Design review of the part built by this model. Coordinates are the model's own, in mm. A direction names the side the tool comes from. Round coordinates to 2 decimals unless told otherwise and drop trailing zeros. Write each loop counter-clockwise with the first axis right and the second up, starting at its lowest first coordinate (ties: lowest second). Pieces come first, ordered by that corner, then holes. Notation, with made-up numbers: M 0.25,-12.5 L 47.25,-12.5 A14 cw 47.25,13.5 Z; hole C 7,-27.5 d8. An arc over 180 degrees is marked long. One line per question, with ' | ' between items. Start each with the question number.
Item 1: Add section D-D, the plane z = 5. State the section outline as (x, y) points.
Item 2: Add section C-C, the plane z = 28.5. State the section outline as (x, y) points.
Item 3: Draft analysis for pull direction Z (two halves, no side actions). For faces 5 (the face through (60, 99, 20)), 6 (the face through (39.08, 42.535, 22.365)), 7 (the face through (21.6, 99.5, 2)), 8 (the face through (-1, 55, 0)), state which applies: released by +Z, released by -Z, zero draft, split by the parting line, or undercut.
Item 4: For L1, parallel to Z at x = -15.5, y = 3.8; L2, parallel to X at y = 100.4, z = 5; L3, parallel to Y at x = 45, z = 11, list the stretches that pass through material, from the lowest coordinate up.
Item 5: Machinability: for faces 1 (the face through (0, 20, 20)), 2 (the face through (3.57, 42.46, 4.35)), 3 (the face through (54.474, 99.535, 4.609)), 4 (the face through (30, 97, 20)), which of the approach directions +Z, -Z, +X, -X, +Y, -Y give a long, thin tool a straight path to every point of the face, cutting with its end or side? Answer none if there is none.
Item 6: Add section A-A, the plane x = 6.5. State the section outline as (y, z) points, and give its area (3 significant figures).
Item 7: Insertion check: pin 1 Ø9.5 at (x, z) = (36.5, 20) entering from +Y; pin 2 Ø4 at (x, z) = (-15.5, 11.5) entering from -Y; pin 3 Ø10 at (x, z) = (16, 6.5) entering from -Y; pin 4 Ø13.5 at (x, z) = (-19, 18) entering from +Y. Each pin has a flat end and moves straight along its axis. Give the tip position at first contact, or say it passes through.
Item 8: Add section B-B, the plane x = 36.5. State the section outline as (y, z) points.
```python
from build123d import *

# Parameters (mm, degrees)
SALIENTE_EXTRUIR1_DEPTH = 40
CORTAR_EXTRUIR1_REACH   = 122.868
CROQUIS2_R              = 3.5
CORTAR_EXTRUIR4_START   = -62
CROQUIS3_R              = 3
CORTAR_EXTRUIR4_DEPTH   = 5
CORTAR_EXTRUIR3_REACH   = 93.918
CROQUIS4_R              = 2.5
CROQUIS4_R_2            = 3.5
CORTAR_EXTRUIR5_REACH   = 126.916
CROQUIS5_R              = 3


with BuildPart() as part:
    # Croquis1 → Saliente-Extruir1 (new body)
    with BuildSketch(Plane.XY):
        Polygon((0, 0), (0, 40), (60, 40), (60, 45), (0, 45), (0, 97), (60, 97), (60, 102), (-7, 102), (-7, 5), (-24, 5), (-24, 0), align=None)
    extrude(amount=SALIENTE_EXTRUIR1_DEPTH)

    # Croquis2 → Cortar-Extruir1 (cut, up to next)
    with BuildSketch(Plane(origin=(0, 5, 0), x_dir=(1, 0, 0), z_dir=(0, 1, 0)), mode=Mode.PRIVATE) as cortar_extruir1_sk1:
        with Locations(Location((-15.5, -11.5, 0), (0, 0, 180))):
            Circle(CROQUIS2_R)
    cortar_extruir1_tool1 = extrude(cortar_extruir1_sk1.sketch, amount=-CORTAR_EXTRUIR1_REACH, mode=Mode.PRIVATE) & part.part
    # Croquis2 → Cortar-Extruir1 (cut, up to next)
    with BuildSketch(Plane(origin=(0, 5, 0), x_dir=(1, 0, 0), z_dir=(0, 1, 0)), mode=Mode.PRIVATE) as cortar_extruir1_sk2:
        with Locations(Location((-15.5, -28.5, 0), (0, 0, 180))):
            Circle(CROQUIS2_R)
    cortar_extruir1_tool2 = extrude(cortar_extruir1_sk2.sketch, amount=-CORTAR_EXTRUIR1_REACH, mode=Mode.PRIVATE) & part.part
    add(cortar_extruir1_tool1.solids().sort_by_distance((-15.5, 5, 11.5))[0], mode=Mode.SUBTRACT)
    add(cortar_extruir1_tool2.solids().sort_by_distance((-15.5, 5, 28.5))[0], mode=Mode.SUBTRACT)

    # Croquis3 → Cortar-Extruir4 (cut)
    with BuildSketch(Plane(origin=(0, 102, 0), x_dir=(1, 0, 0), z_dir=(0, 1, 0)).offset(CORTAR_EXTRUIR4_START)):
        with Locations(Location((6.5, -5, 0), (0, 0, 270))):
            Circle(CROQUIS3_R)
        with Locations(Location((36.5, -5, 0), (0, 0, 270))):
            Circle(CROQUIS3_R)
        with Locations(Location((6.5, -35, 0), (0, 0, 270))):
            Circle(CROQUIS3_R)
        with Locations(Location((36.5, -35, 0), (0, 0, 270))):
            Circle(CROQUIS3_R)
    extrude(amount=CORTAR_EXTRUIR4_DEPTH, mode=Mode.SUBTRACT)

    # Croquis4 → Cortar-Extruir3 (cut, up to next)
    with BuildSketch(Plane(origin=(0, 45, 0), x_dir=(1, 0, 0), z_dir=(0, 1, 0)), mode=Mode.PRIVATE) as cortar_extruir3_sk1:
        with Locations(Location((21.5, -20, 0), (0, 0, 180))):
            Circle(CROQUIS4_R)
    cortar_extruir3_tool1 = extrude(cortar_extruir3_sk1.sketch, amount=-CORTAR_EXTRUIR3_REACH, mode=Mode.PRIVATE) & part.part
    # Croquis4 → Cortar-Extruir3 (cut, up to next)
    with BuildSketch(Plane(origin=(0, 45, 0), x_dir=(1, 0, 0), z_dir=(0, 1, 0)), mode=Mode.PRIVATE) as cortar_extruir3_sk2:
        with Locations(Location((36.5, -20, 0), (0, 0, 180))):
            Circle(CROQUIS4_R_2)
    cortar_extruir3_tool2 = extrude(cortar_extruir3_sk2.sketch, amount=-CORTAR_EXTRUIR3_REACH, mode=Mode.PRIVATE) & part.part
    add(cortar_extruir3_tool1.solids().sort_by_distance((21.5, 45, 20))[0], mode=Mode.SUBTRACT)
    add(cortar_extruir3_tool2.solids().sort_by_distance((36.5, 45, 20))[0], mode=Mode.SUBTRACT)

    # Croquis5 → Cortar-Extruir5 (cut, up to next)
    with BuildSketch(Plane(origin=(0, 102, 0), x_dir=(1, 0, 0), z_dir=(0, 1, 0)), mode=Mode.PRIVATE) as cortar_extruir5_sk1:
        with Locations(Location((21.5, -5, 0), (0, 0, 270))):
            Circle(CROQUIS5_R)
    cortar_extruir5_tool1 = extrude(cortar_extruir5_sk1.sketch, amount=-CORTAR_EXTRUIR5_REACH, mode=Mode.PRIVATE) & part.part
    # Croquis5 → Cortar-Extruir5 (cut, up to next)
    with BuildSketch(Plane(origin=(0, 102, 0), x_dir=(1, 0, 0), z_dir=(0, 1, 0)), mode=Mode.PRIVATE) as cortar_extruir5_sk2:
        with Locations(Location((51.5, -5, 0), (0, 0, 270))):
            Circle(CROQUIS5_R)
    cortar_extruir5_tool2 = extrude(cortar_extruir5_sk2.sketch, amount=-CORTAR_EXTRUIR5_REACH, mode=Mode.PRIVATE) & part.part
    # Croquis5 → Cortar-Extruir5 (cut, up to next)
    with BuildSketch(Plane(origin=(0, 102, 0), x_dir=(1, 0, 0), z_dir=(0, 1, 0)), mode=Mode.PRIVATE) as cortar_extruir5_sk3:
        with Locations(Location((21.5, -35, 0), (0, 0, 270))):
            Circle(CROQUIS5_R)
    cortar_extruir5_tool3 = extrude(cortar_extruir5_sk3.sketch, amount=-CORTAR_EXTRUIR5_REACH, mode=Mode.PRIVATE) & part.part
    # Croquis5 → Cortar-Extruir5 (cut, up to next)
    with BuildSketch(Plane(origin=(0, 102, 0), x_dir=(1, 0, 0), z_dir=(0, 1, 0)), mode=Mode.PRIVATE) as cortar_extruir5_sk4:
        with Locations(Location((51.5, -35, 0), (0, 0, 270))):
            Circle(CROQUIS5_R)
    cortar_extruir5_tool4 = extrude(cortar_extruir5_sk4.sketch, amount=-CORTAR_EXTRUIR5_REACH, mode=Mode.PRIVATE) & part.part
    # Croquis5 → Cortar-Extruir5 (cut, up to next)
    with BuildSketch(Plane(origin=(0, 102, 0), x_dir=(1, 0, 0), z_dir=(0, 1, 0)), mode=Mode.PRIVATE) as cortar_extruir5_sk5:
        with Locations(Location((36.5, -20, 0), (0, 0, 270))):
            Circle(CROQUIS5_R)
    cortar_extruir5_tool5 = extrude(cortar_extruir5_sk5.sketch, amount=-CORTAR_EXTRUIR5_REACH, mode=Mode.PRIVATE) & part.part
    add(cortar_extruir5_tool1.solids().sort_by_distance((21.5, 102, 5))[0], mode=Mode.SUBTRACT)
    add(cortar_extruir5_tool2.solids().sort_by_distance((51.5, 102, 5))[0], mode=Mode.SUBTRACT)
    add(cortar_extruir5_tool3.solids().sort_by_distance((21.5, 102, 35))[0], mode=Mode.SUBTRACT)
    add(cortar_extruir5_tool4.solids().sort_by_distance((51.5, 102, 35))[0], mode=Mode.SUBTRACT)
    add(cortar_extruir5_tool5.solids().sort_by_distance((36.5, 102, 20))[0], mode=Mode.SUBTRACT)


solid = part.part
```
Computed values:
1) outline: M -24,0 L 0,0 L 0,40 L 3.5,40 L 3.5,45 L 0,45 L 0,97 L 18.5,97 L 18.5,102 L -7,102 L -7,5 L -24,5 Z; M 9.5,40 L 33.5,40 L 33.5,45 L 9.5,45 Z; M 24.5,97 L 48.5,97 L 48.5,102 L 24.5,102 Z; M 39.5,40 L 60,40 L 60,45 L 39.5,45 Z; M 54.5,97 L 60,97 L 60,102 L 54.5,102 Z
2) outline: M -24,0 L -19,0 L -19,5 L -24,5 Z; M -12,0 L 0,0 L 0,40 L 60,40 L 60,45 L 0,45 L 0,97 L 60,97 L 60,102 L -7,102 L -7,5 L -12,5 Z
3) face 5: zero draft | face 6: undercut | face 7: undercut | face 8: released by -Z
4) L1: z = 0 to 8, 15 to 25, 32 to 40 | L2: x = -7 to 18.5, 24.5 to 48.5, 54.5 to 60 | L3: y = 40 to 45, 97 to 102
5) face 1: +Z, -Z, +X, -Y | face 2: -Y | face 3: +Y | face 4: +Z, -Z, +X
6) outline: M 40,0 L 45,0 L 45,2 L 40,2 Z; M 40,8 L 45,8 L 45,32 L 40,32 Z; M 40,38 L 45,38 L 45,40 L 40,40 Z; M 97,0 L 102,0 L 102,40 L 97,40 Z | area: 340 mm^2
7) pin 1: stops at y = 102 | pin 2: passes through | pin 3: stops at y = 40 | pin 4: stops at y = 5
8) outline: M 40,0 L 45,0 L 45,2 L 40,2 Z; M 40,8 L 45,8 L 45,16.5 L 40,16.5 Z; M 40,23.5 L 45,23.5 L 45,32 L 40,32 Z; M 40,38 L 45,38 L 45,40 L 40,40 Z; M 97,0 L 102,0 L 102,17 L 97,17 Z; M 97,23 L 102,23 L 102,40 L 97,40 Z
